from build123d import *

# Parameters (mm, degrees)
SKETCH1_W                               = 64
SKETCH1_H                               = 36
BOSS_EXTRUDE1_DEPTH                     = 16
CUT_EXTRUDE1_DEPTH                      = 22
SKETCH3_R                               = 6
CUT_EXTRUDE2_DEPTH                      = 24
SKETCH4_W                               = 16
SKETCH4_H                               = 9
BOSS_EXTRUDE3_DEPTH                     = 32
F_6_0MM_DOWEL_HOLE1_D                   = 6
F_6_0MM_DOWEL_HOLE1_DEPTH               = 16
F_6_0MM_DOWEL_HOLE1_TIP                 = 1.802581857
CBORE_FOR_M6_HEX_HEAD_BOLT2_D           = 6
CBORE_FOR_M6_HEX_HEAD_BOLT2_DEPTH       = 13
CBORE_FOR_M6_HEX_HEAD_BOLT2_CBORE_D     = 10
CBORE_FOR_M6_HEX_HEAD_BOLT2_CBORE_DEPTH = 5
CBORE_FOR_M6_HEX_HEAD_BOLT2_TIP         = 1.802581857


with BuildPart() as part:
    # Sketch1 → Boss-Extrude1 (new, symmetric)
    with BuildSketch(Plane.XY):
        Rectangle(SKETCH1_W, SKETCH1_H)
    extrude(amount=BOSS_EXTRUDE1_DEPTH, both=True)

    # Sketch2 → Cut-Extrude1 (cut)
    with BuildSketch(Plane.XY.offset(16)):
        with BuildLine():
            Line((-32, -8), (-27.499996562, -8))
            ThreePointArc((-27.499996562, -8), (-26.084327344, -7.644972715), (-25.003725591, -6.663920443))
            Line((-25.003725591, -6.663920443), (-13.313445176, 10.874242365))
            ThreePointArc((-13.313445176, 10.874242365), (-0.000751694, 17.999999982), (13.312611277, 10.875493281))
            Line((13.312611277, 10.875493281), (25.007578247, -6.666128828))
            ThreePointArc((25.007578247, -6.666128828), (26.086521715, -7.646142127), (27.500003403, -8.001971569))
            Line((27.500003403, -8.001971569), (32, -8.007505757))
            Line((32, -8.007505757), (36.662231921, -8.007505757))
            Line((36.662231921, -8.007505757), (36.662231921, 30.154585716))
            Line((36.662231921, 30.154585716), (-48.36652886, 30.154585716))
            Line((-48.36652886, 30.154585716), (-48.36652886, -8))
            Line((-48.36652886, -8), (-32, -8))
        make_face()
    extrude(amount=-CUT_EXTRUDE1_DEPTH, mode=Mode.SUBTRACT)

    # Sketch3 → Cut-Extrude2 (cut)
    with BuildSketch(Plane.XY.offset(16)):
        with Locations((0, 2)):
            Circle(SKETCH3_R)
    extrude(amount=-CUT_EXTRUDE2_DEPTH, mode=Mode.SUBTRACT)

    # Sketch4 → Boss-Extrude3 (add)
    with BuildSketch(Plane.XY.offset(16)):
        with Locations((0, -22.5)):
            Rectangle(SKETCH4_W, SKETCH4_H)
    extrude(amount=-BOSS_EXTRUDE3_DEPTH)

    # Ø6.0mm Dowel Hole1
    with Locations(Plane(origin=(0, -27, 8), x_dir=(0, 0, -1), z_dir=(0, -1, 0))):
        with Locations((0, 0), (16, 0)):
            Hole(F_6_0MM_DOWEL_HOLE1_D / 2, depth=F_6_0MM_DOWEL_HOLE1_DEPTH)
            with Locations((0, 0, -(F_6_0MM_DOWEL_HOLE1_DEPTH + F_6_0MM_DOWEL_HOLE1_TIP / 2))):  # 118° drill point
                Cone(0, F_6_0MM_DOWEL_HOLE1_D / 2, F_6_0MM_DOWEL_HOLE1_TIP, mode=Mode.SUBTRACT)

    # CBORE for M6 Hex Head Bolt2
    with Locations(Plane(origin=(0, 18, 0), x_dir=(1, 0, 0), z_dir=(0, 1, 0))):
        with Locations((0, -4)):
            CounterBoreHole(CBORE_FOR_M6_HEX_HEAD_BOLT2_D / 2, CBORE_FOR_M6_HEX_HEAD_BOLT2_CBORE_D / 2, CBORE_FOR_M6_HEX_HEAD_BOLT2_CBORE_DEPTH, depth=CBORE_FOR_M6_HEX_HEAD_BOLT2_DEPTH)
            with Locations((0, 0, -(CBORE_FOR_M6_HEX_HEAD_BOLT2_DEPTH + CBORE_FOR_M6_HEX_HEAD_BOLT2_TIP / 2))):  # 118° drill point
                Cone(0, CBORE_FOR_M6_HEX_HEAD_BOLT2_D / 2, CBORE_FOR_M6_HEX_HEAD_BOLT2_TIP, mode=Mode.SUBTRACT)


solid = part.part
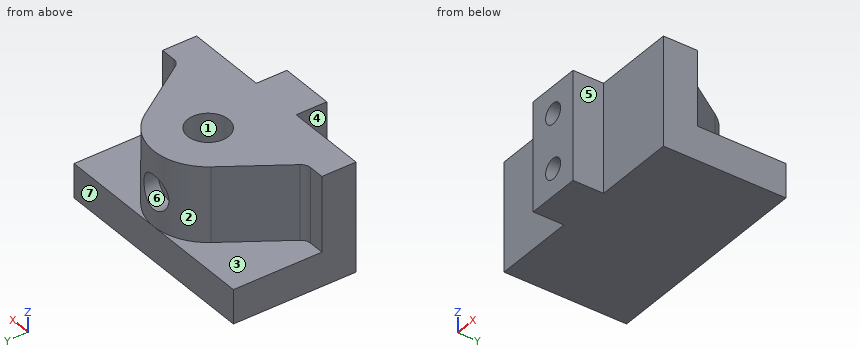
Could you check a few things on this model? Use its own coordinates, in mm. Face numbers are marked on the shaded views. A direction names the side the tool comes from. Give positions to 0.01 mm unless a question says otherwise; leave off trailing zeros. Order: outer loops, then holes, each group sorted by start corner. A loop starts at its lowest first (then second) coordinate and runs counter-clockwise, first axis right, second up. Notation, with made-up numbers: (78.5, 75) - (110.5, 75) arc R34 cw to (110.5, 109) - close; hole circle Ø11 at (81.25, -35). An arc over 180 degrees is marked (long way). Return JSON: item names as keys, results as strings. Group by question number.
Q1. Suppose I cut it at C-C, the plane y = 2. Please give me the cut outline in (x, z), and give its area (3 significant figures).
Q2. Will these pins go through, and if not, where does the flat tip stop? pin 1 Ø7 at (x, z) = (19, -2) entering from -Y; pin 2 Ø4.5 at (y, z) = (-22, -6.5) entering from +X; pin 3 Ø3 at (x, y) = (14, -21) entering from -Z; pin 4 Ø3 at (x, z) = (-2, 2) entering from +Y.
Q3. Thinking about a two-plate mould opening in X: for the marked faces 5, 6 and 7, which applies, pulls with the +X half, pulls with the -X half, needs draft (parallel to the pull), parting line crosses it, or undercut?
Q4. Suppose I cut it at D-D, the plane z = 4. Please give me the cut outline in (x, y).
Q5. Suppose I cut it at A-A, the plane y = -12. Please give me the cut outline in (x, z).
Q6. Please list where these lines run through material, in increasing order: line 1 along Z through (x, y) = (0, -23); line 2 along X through (y, z) = (-18.5, 8); line 3 along Z through (x, y) = (0, 11.65). Write a range as [from, to].
Q7. Which directions (+Z, -Z, +X, -X, +Y, -Y) give clear straight access to the entire face, cutting with the end or side of a thin tool? Please do the marked faces 1, 2, 3 and 4.
Q8. Suppose I cut it at B-B, the plane z = -4. Please give me the cut outline in (x, y).
Resolved:
{
 "1": {"outline": "(-32, -16) - (32, -16) - (32, -6) - (19.23, -6) - (19.23, 16) - (6, 16) - (6, -8) - (-6, -8) - (-6, 16) - (-19.23, 16) - (-19.23, -6) - (-32, -6) - close", "area": "1,200 mm2"},
 "2": {"pin 1": "stops at y = -18", "pin 2": "stops at x = 8", "pin 3": "passes through", "pin 4": "stops at y = 13"},
 "3": {"face 5": "pulls with the +X half", "face 6": "undercut", "face 7": "needs draft"},
 "4": {"outline": "(-32, -18) - (-8, -18) - (-8, -27) - (8, -27) - (8, -18) - (32, -18) - (32, -8.01) - (27.5, -8) arc R3 cw to (25.01, -6.67) - (13.31, 10.88) arc R16 ccw to (5, 17.2) - (5, 13) - (3, 13) - (3, 7.2) arc R6 cw (long way) to (-3, 7.2) - (-3, 13) - (-5, 13) - (-5, 17.2) arc R16 ccw to (-13.31, 10.87) - (-25, -6.66) arc R3 cw to (-27.5, -8) - (-32, -8) - close"},
 "5": {"outline": "(-32, -16) - (32, -16) - (32, 16) - (-32, 16) - close; hole circle Ø6 at (0, -8); hole circle Ø6 at (0, 8)"},
 "6": {"line 1": "z = [-16, -11], [-5, 5], [11, 16]", "line 2": "x = [-8, -3], [3, 8]", "line 3": "z = [-16, 1], [7, 16]"},
 "7": {"face 1": "+Z", "face 2": "+Z, +Y", "face 3": "+Z, -X, +Y", "face 4": "+Z, -Z, -X, -Y"},
 "8": {"outline": "(-32, -18) - (-8, -18) - (-8, -27) - (8, -27) - (8, -18) - (32, -18) - (32, -8.01) - (27.5, -8) arc R3 cw to (25.01, -6.67) - (13.31, 10.88) arc R16 ccw to (-13.31, 10.87) - (-25, -6.66) arc R3 cw to (-27.5, -8) - (-32, -8) - close; hole circle Ø12 at (0, 2)"}
}
